```python
from build123d import *

# Parameters (mm, degrees)
PAD_DEPTH    = 92
POCKET_DEPTH = 100


with BuildPart() as part:
    # Sketch → Pad (new body)
    with BuildSketch(Plane.XY):
        Polygon((-107.002418, 5.939697), (-23.563818, 89.378297), (-28.315576, 94.130055), (-27.127636, 95.317994), (-20, 88.190358), (0, 0), (-105.814479, 0), (-119.051518, 13.237039), (-114.29976, 17.988797), (-113.111821, 16.800857), (-115.4877, 14.424978), align=None)
        Polygon((-22.80842, 85.381938), (-104.830358, 3.36), (-4.207307, 3.36), align=None, mode=Mode.SUBTRACT)
    extrude(amount=PAD_DEPTH)

    # Sketch001 (on Face1 of Pad) → Pocket (cut, symmetric)
    with BuildSketch(Plane(origin=(-56.471058, 56.471058, 0), x_dir=(-0.707107, -0.707107, 0), z_dir=(-0.707107, 0.707107, 0))):
        Polygon((85.037769, 66), (31.462136, 66), (21.462136, 83), (-46.537864, 92), (-46.537864, 107.253265), (85.037769, 107.253265), align=None)
    extrude(amount=POCKET_DEPTH, both=True, mode=Mode.SUBTRACT)


solid = part.part
```
Here's how the part is built. I have some questions about the finished solid (model axes, mm). A direction names the side the tool comes from. Give positions to 0.01 mm unless a question says otherwise; leave off trailing zeros. Loops run counter-clockwise (first coordinate to the right, second up) from the corner with the lowest first, then second, coordinate; pieces in that order, holes last. Notation, with made-up numbers: (-13.5, 27.5) -> (13.5, 27.5) arc R18 cw to (13.5, 51.5) -> close; hole circle Ø7 at (78.5, 78.25). An arc over 180 degrees is marked (long way). Use one line per item in the form item = value. Start each with the question number.
1) For P1, Ø10.5, axis at x = -94.5, y = 22.5, coming from the +Z side; P2, Ø2, axis at y = 44.5, z = 10.5, coming from the +X side (3 decimals); P3, Ø8, axis at y = 23.5, z = 24, coming from the -X side, each with a flat end and sliding along its axis, tell me the tip position at first contact or that it passes through.
2) Imagine slicing it at D-D (y = 61.5). Please give me the cut outline in (x, z).
3) Please list where these lines run through material, in increasing order: line 1 along X through (y, z) = (8.5, 58.5); line 2 along Y through (x, z) = (-33, 29.5); line 3 along X through (y, z) = (67, 10.5).
4) Thinking about a two-plate mould opening in X: for faces 5 (the face through (-63.245, 44.945, 35.018)), 6 (the face through (-39.144, 1.688, 74.46)), 7 (the face through (-23.5, 90.6, 92)), which applies, +X half, -X half, draft (parallel to the pull), parting line (faces both ways), or undercut?
5) Which directions (+Z, -Z, +X, -X, +Y, -Y) give clear straight access to the entire face, cutting with the end or side of a thin tool? Please do faces 1 (the face through (-85, 3, 66)), 2 (the face through (-25.906, 91.721, 45.356)), 3 (the face through (-23.61, 91.8, 45.36)), 4 (the face through (-111.3, 10.24, 32.54)).
6) Imagine slicing it at B-B (x = -86). Please give me the cut outline in (y, z).
7) Imagine slicing it at A-A (y = 8). Please give me the cut outline in (x, z).
8) Imagine slicing it at C-C (z = 7). Please give me the cut outline in (x, y).
Check values:
q1.P1 = 66
q1.P2 = -9.865
q1.P3 = -93.44
q2.outline = (-51.44, 0) -> (-46.69, 0) -> (-46.69, 87.23) -> (-51.44, 86.78) -> close; (-17.39, 0) -> (-13.95, 0) -> (-13.95, 90.29) -> (-17.39, 89.97) -> close
q3.line_1 = -114.31 to -109.56, -104.44 to -99.69, -5.37 to -1.93
q3.line_2 = 0 to 3.36, 75.19 to 79.94
q3.line_3 = -45.94 to -41.19, -18.64 to -15.19
q4.face_5 = undercut
q4.face_6 = -X half
q4.face_7 = draft
q5.face_1 = +Z, -X, -Y
q5.face_2 = +Z, -Z, -X
q5.face_3 = +Z, -Z, +X, +Y
q5.face_4 = +Z, -Z
q6.outline = (0, 0) -> (3.36, 0) -> (3.36, 66) -> (0, 66) -> close; (22.19, 0) -> (26.94, 0) -> (26.94, 66) -> (22.19, 66) -> close
q7.outline = (-113.81, 0) -> (-109.06, 0) -> (-109.06, 66) -> (-113.81, 66) -> close; (-104.94, 0) -> (-100.19, 0) -> (-100.19, 66) -> (-104.94, 66) -> close; (-5.26, 0) -> (-1.81, 0) -> (-1.81, 86.42) -> (-5.26, 86.1) -> close
q8.outline = (-119.05, 13.24) -> (-105.81, 0) -> (0, 0) -> (-20, 88.19) -> (-27.13, 95.32) -> (-28.32, 94.13) -> (-23.56, 89.38) -> (-107, 5.94) -> (-115.49, 14.42) -> (-113.11, 16.8) -> (-114.3, 17.99) -> close; hole (-104.83, 3.36) -> (-4.21, 3.36) -> (-22.81, 85.38) -> close
